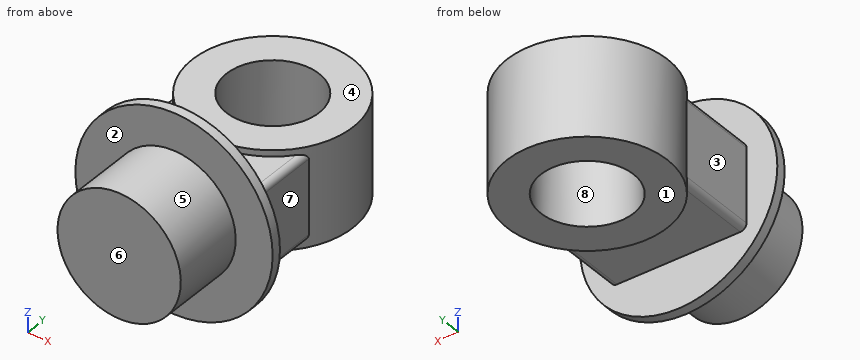
from build123d import *

# Parameters (mm, degrees)
IZIM2_R                          = 100
Y_KSEKLIK_EKSTR_ZYON1_DEPTH      = 120
IZIM3_R                          = 160
Y_KSEKLIK_EKSTR_ZYON2_DEPTH      = 16
IZIM4_R                          = 130
IZIM4_R_2                        = 75
Y_KSEKLIK_EKSTR_ZYON3_DEPTH      = 90
Y_KSEKLIK_EKSTR_ZYON4_REACH      = 402.125
Y_KSEKLIK_EKSTR_ZYON4_END_RADIUS = 130
SKETCH1_R                        = 137.362830178
SKETCH1_R_2                      = 73.465354293
CUT_EXTRUDE1_DEPTH               = 20
FILLET1_R                        = 10
FILLET2_R                        = 10


with BuildPart() as part:
    # izim2 → Y_kseklik-Ekstr_zyon1 (new body)
    with BuildSketch(Plane(origin=(0, 0, 0), x_dir=(1, 0, 0), z_dir=(0, 1, 0))):
        with Locations(Location((0, 0, 0), (0, 0, 270))):
            Circle(IZIM2_R)
    extrude(amount=Y_KSEKLIK_EKSTR_ZYON1_DEPTH)

    # izim3 → Y_kseklik-Ekstr_zyon2 (add)
    with BuildSketch(Plane(origin=(0, 120, 0), x_dir=(1, 0, 0), z_dir=(0, 1, 0))):
        with Locations(Location((0, 0, 0), (0, 0, 270))):
            Circle(IZIM3_R)
    extrude(amount=Y_KSEKLIK_EKSTR_ZYON2_DEPTH)



with BuildPart() as body_2:
    # izim4 → Y_kseklik-Ekstr_zyon3 (new, symmetric)
    with BuildSketch(Plane.XY):
        with Locations(Location((0, 336, 0), (0, 0, 180))):
            Circle(IZIM4_R)
        with Locations(Location((0, 336, 0), (0, 0, 180))):
            Circle(IZIM4_R_2, mode=Mode.SUBTRACT)
    extrude(amount=Y_KSEKLIK_EKSTR_ZYON3_DEPTH, both=True)


with BuildPart() as part_1:
    add(part.part)

    add(body_2.part)  # Y_kseklik-Ekstr_zyon4 merges body 2
    # Y_kseklik-Ekstr_zyon4: up to this cylinder (the profile starts outside it)
    y_kseklik_ekstr_zyon4_end = Plane(origin=(0, 336, -10), z_dir=(0, 0, -1)) * Cylinder(Y_KSEKLIK_EKSTR_ZYON4_END_RADIUS, 1065.25, mode=Mode.PRIVATE)
    # izim6 → Y_kseklik-Ekstr_zyon4 (add, up to the surface)
    with BuildSketch(Plane(origin=(0, 136, 0), x_dir=(1, 0, 0), z_dir=(0, 1, 0)), mode=Mode.PRIVATE) as y_kseklik_ekstr_zyon4_sk1:
        Polygon((107.277662826, -60), (110, -60), (110, 80), (-110, 80), (-110, -60), align=None)
    y_kseklik_ekstr_zyon4_tool1 = extrude(y_kseklik_ekstr_zyon4_sk1.sketch, amount=Y_KSEKLIK_EKSTR_ZYON4_REACH, mode=Mode.PRIVATE) - y_kseklik_ekstr_zyon4_end
    add(y_kseklik_ekstr_zyon4_tool1.solids().sort_by_distance((0, 136, -10))[0])

    # Sketch1 → Cut-Extrude1 (cut)
    with BuildSketch(Plane.XY.offset(90)):
        with Locations((0, 334.465354293)):
            Circle(SKETCH1_R)
        with Locations((0, 334.465354293)):
            Circle(SKETCH1_R_2, mode=Mode.SUBTRACT)
    extrude(amount=-CUT_EXTRUDE1_DEPTH, mode=Mode.SUBTRACT)

    # Fillet1
    fillet1_edges = [part_1.edges().sort_by_distance(p)[0] for p in [
        (-110, 201.358983849, 60),
        (110, 201.358983849, 60),
    ]]
    fillet(fillet1_edges, radius=FILLET1_R)

    # Fillet2
    fillet2_edges = [part_1.edges().sort_by_distance(p)[0] for p in [
        (110, 201.358983849, -80),
        (-110, 201.358983849, -80),
    ]]
    fillet(fillet2_edges, radius=FILLET2_R)


solid = part_1.part
Here's how the part is built. I have some questions about the finished solid (model axes, mm). Face numbers are marked on the shaded views. A direction names the side the tool comes from. Round coordinates to 2 decimals unless told otherwise and drop trailing zeros. Order: outer loops, then holes, each group sorted by start corner. A loop starts at its lowest first (then second) coordinate and runs counter-clockwise, first axis right, second up. Notation, with made-up numbers: M -7,60.5 L 8,60.5 A24 cw 8,90.5 Z; hole C 40.5,54 d4. An arc over 180 degrees is marked long. Return JSON: item names as keys, results as strings. Group by question number.
1. On a 3-axis mill with a long thin cutter (end or side, diameter ignored), from which of +Z, -Z, +X, -X, +Y, -Y can I reach the whole of each face in a straight line? I mean the marked faces 1, 2, 3 and 4. Say none if no direction works.
2. If we section it at A-A on x = 0: List the corners of the cut face in (y, z) for me, then the cut area to 3 significant figures.
3. I'm going to push flat-ended pins straight in: pin 1 Ø5 at (y, z) = (89, 56.5) entering from -X; pin 2 Ø4 at (x, z) = (107, 98.5) entering from -Y; pin 3 Ø8 at (y, z) = (258, -27.5) entering from -X. Where does each tip first touch, or does it pass through?
4. If we section it at C-C on z = 0: List the corners of the cut face in (x, y) for me, then the cut area to 3 significant figures.
5. Please list where these lines run through material, in increasing order: probe 1 along X at (y, z) = (336, -40); probe 2 along Y at (x, z) = (0, -25.5); probe 3 along Y at (x, z) = (25, 64.5).
6. If we mould it in two halves opening along Y, with no side actions, what happens to the marked faces 5, 6, 7 and 8? For each: pulls with the +Y half, pulls with the -Y half, needs draft (parallel to the pull), parting line crosses it, or undercut.
7. If we section it at B-B on y = 336: List the corners of the cut face in (x, z) for me, then the cut area to 3 significant figures.
8. If we section it at D-D on y = 220.5: List the corners of the cut face in (x, z) for me, then the cut area to 3 significant figures.
Reply:
{
 "1": {"face 1": "-Z, +X, -X, +Y", "face 2": "-Y", "face 3": "+Z, -Z, -X", "face 4": "+Z, +X, -X, +Y"},
 "2": {"outline": "M 0,-100 L 120,-100 L 120,-160 L 136,-160 L 136,-80 L 206,-80 L 206,-90 L 261,-90 L 261,70 L 206,70 L 206,60 L 136,60 L 136,160 L 120,160 L 120,100 L 0,100 Z; M 411,-90 L 466,-90 L 466,70 L 411,70 Z", "area": "56,500 mm^2"},
 "3": {"pin 1": "x = -84.17", "pin 2": "y = 120", "pin 3": "x = -110"},
 "4": {"outline": "M -160,120 L -100,120 L -100,0 L 100,0 L 100,120 L 160,120 L 160,136 L 110,136 L 110,266.72 A130 ccw long -110,266.72 L -110,136 L -160,136 Z; hole C 0,336 d150", "area": "83,900 mm^2"},
 "5": {"probe 1": "-130 to -75, 75 to 130", "probe 2": "0 to 261, 411 to 466", "probe 3": "0 to 136, 208.43 to 265.29, 406.71 to 463.57"},
 "6": {"face 5": "needs draft", "face 6": "pulls with the -Y half", "face 7": "undercut", "face 8": "undercut"},
 "7": {"outline": "M -130,-90 L -75,-90 L -75,70 L -130,70 Z; M 75,-90 L 130,-90 L 130,70 L 75,70 Z", "area": "17,600 mm^2"},
 "8": {"outline": "M -110,-70 A10 ccw -100,-80 L -59.66,-80 L -59.66,-90 L 59.66,-90 L 59.66,-80 L 100,-80 A10 ccw 110,-70 L 110,50 A10 ccw 100,60 L 59.66,60 L 59.66,70 L -59.66,70 L -59.66,60 L -100,60 A10 ccw -110,50 Z", "area": "33,100 mm^2"}
}
